```python
from build123d import *

# Parameters (mm, degrees)
PAD_DEPTH = 5


with BuildPart() as part:
    # Sketch001 → Pad (new body)
    with BuildSketch(Plane.XY):
        with BuildLine():
            Line((-3.5, 4.5), (3.25, 4.25))
            ThreePointArc((5.375, 3.680608), (4.349981, 4.105185), (3.25, 4.25))
            ThreePointArc((4.375, 1.948557), (5.741025, 2.314583), (5.375, 3.680608))
            ThreePointArc((4.375, 1.948557), (1, 0), (4.375, -1.948557))
            ThreePointArc((5.375, -3.680608), (5.741025, -2.314583), (4.375, -1.948557))
            ThreePointArc((3.25, -4.25), (4.349981, -4.105185), (5.375, -3.680608))
            Line((-3.5, -4.5), (3.25, -4.25))
            ThreePointArc((-5.75, -3.897114), (-4.664686, -4.346666), (-3.5, -4.5))
            ThreePointArc((-4.75, -2.165064), (-6.116025, -2.531089), (-5.75, -3.897114))
            ThreePointArc((-4.75, -2.165064), (-1, 0), (-4.75, 2.165064))
            ThreePointArc((-5.75, 3.897114), (-6.116025, 2.531089), (-4.75, 2.165064))
            ThreePointArc((-3.5, 4.5), (-4.664686, 4.346666), (-5.75, 3.897114))
        make_face()
    extrude(amount=PAD_DEPTH)


solid = part.part
```
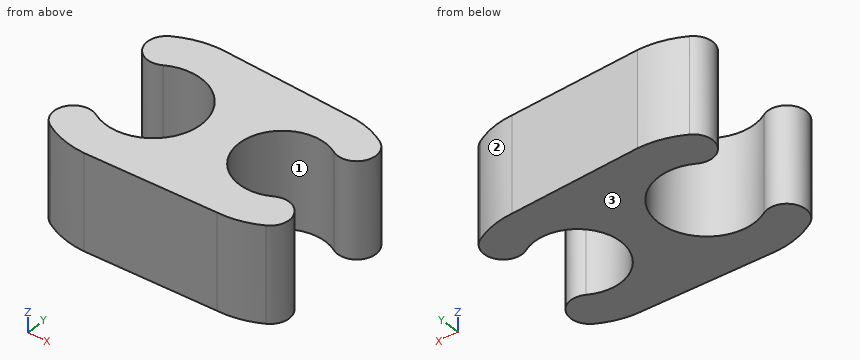
Verification items for the finished model (mm, model axes). Face numbers are marked on the shaded views. Round coordinates to 2 decimals unless told otherwise and drop trailing zeros. Order: outer loops, then holes, each group sorted by start corner. A loop starts at its lowest first (then second) coordinate and runs counter-clockwise, first axis right, second up. Notation, with made-up numbers: (49, -10.75) - (56, -10.75) arc R35 ccw to (56, 28.25) - close; hole circle Ø6 at (-26, 88). An arc over 180 degrees is marked (long way). Use CSV: the item, a comma, the result in double quotes. Start each with the question number.
1) Go/stop test with a flat-tipped pin: P1, Ø2, axis at x = 4.5, z = 3.5, coming from the -Y side. Record where the tip stops, or that it passes through.
2) Section check C-C, the plane z = 3.5. Record the cut outline in (x, y) (3 decimals), plus the area to 3 significant figures.
3) Section check B-B, the plane x = -5.25. Record the cut outline in (y, z).
4) Section check A-A, the plane x = -2.5. Record the cut outline in (y, z).
5) Section check D-D, the plane y = 0. Record the cut outline in (x, z).
6) Thickness scan on L1, parallel to Y at x = 3.25, z = 2.25; L2, parallel to Y at x = -3.5, z = 2.2; L3, parallel to X at y = -0.25, z = 2.9. Record the ranges inside material, lowest first.
7) Mould release check, pull along X, two halves, no side actions. Record for the marked faces 1, 2 and 3: +X half, -X half, draft (parallel to the pull), parting line (faces both ways), or undercut.
Answers:
1,P1,"stops at y = -4.24"
2,outline,"(-5.75, -3.897) arc R4.5 ccw to (-3.5, -4.5) - (3.25, -4.25) arc R4.25 ccw to (5.375, -3.681) arc R1 ccw to (4.375, -1.949) arc R2.25 cw (long way) to (4.375, 1.949) arc R1 ccw to (5.375, 3.681) arc R4.25 ccw to (3.25, 4.25) - (-3.5, 4.5) arc R4.5 ccw to (-5.75, 3.897) arc R1 ccw to (-4.75, 2.165) arc R2.5 cw (long way) to (-4.75, -2.165) arc R1 ccw to start"
2,area,"61.7 mm²"
3,outline,"(-4.15, 0) - (-2.03, 0) - (-2.03, 5) - (-4.15, 5) - close; (2.03, 0) - (4.15, 0) - (4.15, 5) - (2.03, 5) - close"
4,outline,"(-4.46, 0) - (-2.29, 0) - (-2.29, 5) - (-4.46, 5) - close; (2.29, 0) - (4.46, 0) - (4.46, 5) - (2.29, 5) - close"
5,outline,"(-1, 0) - (1, 0) - (1, 5) - (-1, 5) - close"
6,L1,"y = -4.25 to -2.25, 2.25 to 4.25"
6,L2,"y = -4.5 to -2.5, 2.5 to 4.5"
6,L3,"x = -1.01 to 1.01"
7,face 1,"undercut"
7,face 2,"+X half"
7,face 3,"draft"
